Read the model definition and answer for the solid it produces. Units are mm, in the model's axes. A direction names the side the tool comes from. Coordinates: 2 decimals unless noted, no trailing zeros. Loops run counter-clockwise (first coordinate to the right, second up) from the corner with the lowest first, then second, coordinate; pieces in that order, holes last. Notation, with made-up numbers: (-16.75, 37.5) - (42.25, 37.5) arc R11 cw to (42.25, 42.5) - close; hole circle Ø10 at (-5.5, 46). An arc over 180 degrees is marked (long way). Use one line per item in the form item = value. Start each with the question number.
1) Each of these flat-tipped pins is pushed along its axis until it touches: P1, Ø1.9, axis at x = 2, z = 46.5, coming from the -Y side; P2, Ø1, axis at x = 4, y = -28, coming from the +Z side; P3, Ø2, axis at x = 1.5, y = -64.5, coming from the +Z side; P4, Ø8.5, axis at y = 0, z = 0, coming from the -X side. Where does it stop, or does it pass through?
2) A cutting plane is placed at B-B (z = 177.8). Give the vertices of the cut face in (x, y) (3 decimals).
3) Consider line 1 (Y direction, x = 5.5, z = 54.5); line 2 (Y direction, x = 6, z = 0); line 3 (Z direction, x = 1, y = -13). Determine where each line is inside the solid, lowest interval first.
4) Which of the six approach directions +Z, -Z, +X, -X, +Y, -Y give full straight-line access (tool end or side, diameter ignored) to faces 4 (the face through (3.13, 3.57, 66.31)), 5 (the face through (3.131, 22.327, -20.611))?
5) A cutting plane is placed at C-C (y = -39). Give the vertices of the cut face in (x, z), and give its area (3 significant figures).
6) A cutting plane is placed at A-A (x = 1.75). State how many separate pieces and enclosed holes the cut face has, and give its area (3 significant figures).
7) The mould has two halves that part along Y. Classify faces 1 (the face through (3.131, 7.279, -45.548)), 2 (the face through (3.131, 30.834, 14.078)), 3 (the face through (3.131, -8.447, 2.771)): released by +Y, released by -Y, zero draft, split by the parting line, or undercut.
from build123d import *

# Parameters (mm, degrees)
SKETCH1_R           = 4.7625
BOSS_EXTRUDE1_DEPTH = 6.35


with BuildPart() as part:
    # Sketch1 → Boss-Extrude1 (new body)
    with BuildSketch(Plane(origin=(0, 0, 0), x_dir=(0, 0, -1), z_dir=(1, 0, 0))):
        with BuildLine():
            Line((1.456949245, -8.769800391), (51.554431531, -0.446978235))
            ThreePointArc((51.554431531, -0.446978235), (57.919565723, 6.766351601), (52.149062737, 14.463646963))
            Line((52.149062737, 14.463646963), (-11.823304022, 30.413749404))
            ThreePointArc((-11.823304022, 30.413749404), (-14.110305141, 30.837620007), (-16.431916133, 30.979615818))
            Line((-16.431916133, 30.979615818), (-76.842742751, 30.979615818))
            ThreePointArc((-76.842742751, 30.979615818), (-87.163314642, 28.788359771), (-95.703176645, 22.59267061))
            Line((-95.703176645, 22.59267061), (-194.302879657, -86.713577057))
            ThreePointArc((-194.302879657, -86.713577057), (-194.588070452, -87.035958133), (-194.866964637, -87.363801663))
            ThreePointArc((-194.866964637, -87.363801663), (-194.462569451, -91.835682088), (-189.990689026, -91.431286902))
            ThreePointArc((-189.990689026, -91.431286902), (-167.631286902, -89.409310974), (-165.609310974, -111.768713098))
            ThreePointArc((-165.609310974, -111.768713098), (-165.204915788, -116.240593522), (-160.733035363, -115.836198337))
            ThreePointArc((-160.733035363, -115.836198337), (-160.46054239, -115.503015314), (-160.194552833, -115.164617763))
            Line((-160.194552833, -115.164617763), (-72.883126037, -1.843568956))
            ThreePointArc((-72.883126037, -1.843568956), (-66.201418924, 3.623376815), (-57.792742751, 5.579615818))
            Line((-57.792742751, 5.579615818), (-26.042742751, 5.579615818))
            ThreePointArc((-26.042742751, 5.579615818), (-18.752623365, 4.129520913), (-12.572358569, 0))
            Line((-12.572358569, 0), (-6.286179285, -6.286179285))
            ThreePointArc((-6.286179285, -6.286179285), (-2.715227273, -8.465201761), (1.456949245, -8.769800391))
        make_face()
        Circle(SKETCH1_R, mode=Mode.SUBTRACT)
        with Locations((50.305617892, 7.069993529)):
            Circle(SKETCH1_R, mode=Mode.SUBTRACT)
    extrude(amount=BOSS_EXTRUDE1_DEPTH)


solid = part.part
Found:
q1.P1 = 5.58
q1.P2 = 141.79
q1.P3 = 175.17
q1.P4 = through
q2.outline = (0, -85.725) - (6.35, -85.725) - (6.35, -68.419) - (0, -68.419) - close
q3.line_1 = 5.58 to 30.98
q3.line_2 = -8.89 to -4.76, 4.76 to 27.47
q3.line_3 = 81.48 to 127.81
q4.face_4 = +X, -X, -Y
q4.face_5 = -Z, +X, -X, +Y
q5.outline = (0, 101.51) - (6.35, 101.51) - (6.35, 151.26) - (0, 151.26) - close
q5.area = 316 mm^2
q6.separate_pieces = 1
q6.enclosed_holes = 2
q6.area = 9,000 mm^2
q7.face_1 = undercut
q7.face_2 = released by +Y
q7.face_3 = released by -Y
